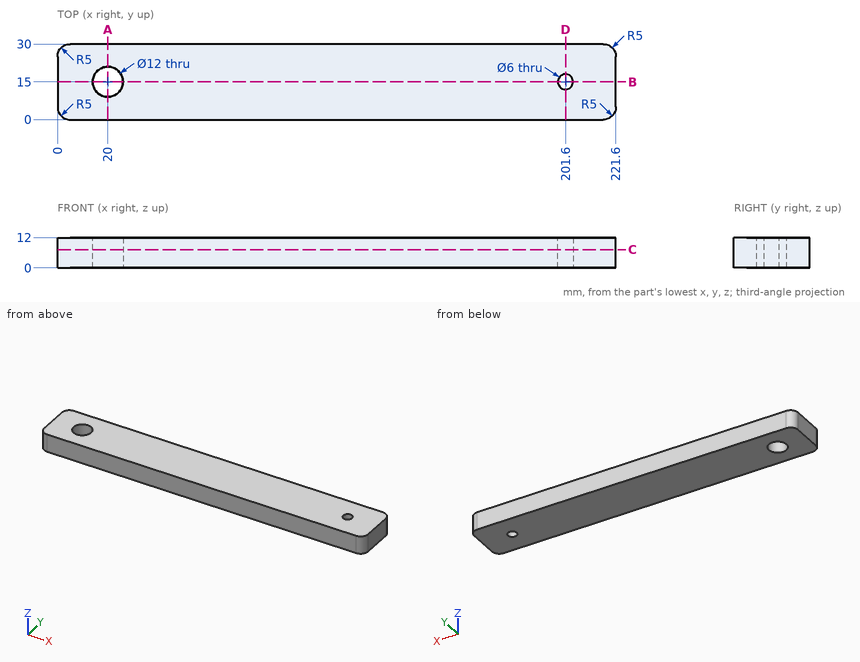
Could you check a few things on this drawing? It's one solid part, dimensions in mm from its lowest x, y, z. Coordinates: 2 decimals unless noted, no trailing zeros. Loops run counter-clockwise (first coordinate to the right, second up) from the corner with the lowest first, then second, coordinate; pieces in that order, holes last. Notation, with made-up numbers: (19, 48.25) - (61, 48.25) arc R26 cw to (61, 79.25) - close; hole circle Ø9 at (58, 65). An arc over 180 degrees is marked (long way). Answer as a JSON object with one key per item and string values. Group by question number.
Item 1: If I drill on L1, parallel to Y at x = 201.6, z = 5.5; L2, parallel to Y at x = 20, z = 2.5; L3, parallel to X at y = 18.5, z = 11.5, over which ranges is the centre line in solid material (lowest first)? Write a range as from..to.
Item 2: If we section it at C-C (z = 7.25): List the corners of the cut face in (x, y) for me.
Item 3: If we section it at B-B (y = 15): List the corners of the cut face in (x, z) for me.
Item 4: For pin 1 (5 mm diameter, centred on x = 201.6, y = 15, fed in from +Z); pin 2 (1 mm diameter, centred on x = 44.5, z = 4.5, fed in from -Y), each with a flat end and sliding along its axis, tell me the tip position at first contact or that it passes through.
Item 5: If we section it at D-D (x = 201.6): List the corners of the cut face in (y, z) for me.
Item 6: If we section it at A-A (x = 20): List the corners of the cut face in (y, z) for me.
Returned:
{
 "1": {"L1": "y = 0..12, 18..30", "L2": "y = 0..9, 21..30", "L3": "x = 0..15.13, 24.87..221.6"},
 "2": {"outline": "(0, 5) arc R5 ccw to (5, 0) - (216.6, 0) arc R5 ccw to (221.6, 5) - (221.6, 25) arc R5 ccw to (216.6, 30) - (5, 30) arc R5 ccw to (0, 25) - close; hole circle Ø12 at (20, 15); hole circle Ø6 at (201.6, 15)"},
 "3": {"outline": "(0, 0) - (14, 0) - (14, 12) - (0, 12) - close; (26, 0) - (198.6, 0) - (198.6, 12) - (26, 12) - close; (204.6, 0) - (221.6, 0) - (221.6, 12) - (204.6, 12) - close"},
 "4": {"pin 1": "passes through", "pin 2": "stops at y = 0"},
 "5": {"outline": "(0, 0) - (12, 0) - (12, 12) - (0, 12) - close; (18, 0) - (30, 0) - (30, 12) - (18, 12) - close"},
 "6": {"outline": "(0, 0) - (9, 0) - (9, 12) - (0, 12) - close; (21, 0) - (30, 0) - (30, 12) - (21, 12) - close"}
}
